Check sheet for the modelled part. Datum: model origin and axes. Units: mm. Face numbers are marked on the shaded views. A direction names the side the tool comes from. Round coordinates to 2 decimals unless told otherwise and drop trailing zeros. Loops run counter-clockwise (first coordinate to the right, second up) from the corner with the lowest first, then second, coordinate; pieces in that order, holes last. Notation, with made-up numbers: M 32.25,-32 L 59.25,-32 A6 ccw 59.25,-28 Z; hole C -22,-33.75 d10. An arc over 180 degrees is marked long. Write item = value, one per line. Start each with the question number.
(1) Go/stop test with flat-tipped pins: P1, Ø3, axis at y = 5, z = 1, coming from the -X side; P2, Ø3, axis at x = -18, z = 1, coming from the +Y side; P3, Ø2, axis at x = -126, z = 2.5, coming from the -Y side. Record where each tip stops, or that it passes through.
(2) Scan lines: L1, parallel to Y at x = -99.5, z = 12; L2, parallel to Z at x = -132, y = 28; L3, parallel to Y at x = -140, z = 0.9. Record each from-to range of solid material in increasing order. Write a range as from..to.
(3) Set-up check for the marked faces 1 and 2: record each of +Z, -Z, +X, -X, +Y, -Y from which the full face is reachable in a straight line by a thin tool's end or side.
(4) Mould release check, pull along X, two halves, no side actions. Record for the marked faces 3 and 4: pulls with the +X half, pulls with the -X half, needs draft (parallel to the pull), parting line crosses it, or undercut.
(5) Cross-section at A-A on x = -72.5. Record the boundary of the cut face in (y, z), plus the area to 3 significant figures.
(6) Cross-section at B-B on x = -127. Record the boundary of the cut face in (y, z).
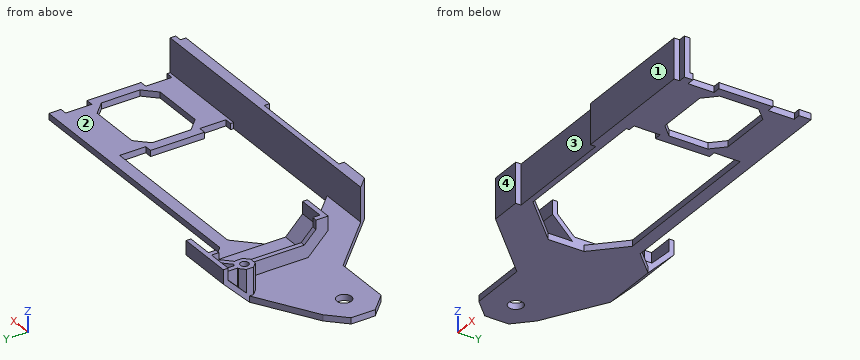
from build123d import *

# Parameters (mm, degrees)
SKETCH4_R            = 3
MAIN_WALL_DEPTH      = 2.5
BASE_DEPTH           = 14
BOSS_EXTRUDE8_DEPTH  = 2
BOSS_EXTRUDE9_DEPTH  = 11
BOSS_EXTRUDE15_DEPTH = 12.5
BOSS_EXTRUDE13_REACH = 169.888
SKETCH19_R           = 1.7
CUT_EXTRUDE1_DEPTH   = 7


with BuildPart() as part:
    # Sketch4 → Main Wall (new body)
    with BuildSketch(Plane.XY):
        Polygon((-97, 59.3), (-113.5, 59.3), (-120.5, 59.3), (-144.970562748, 45), (-152, 37.970562748), (-152, 28.029437252), (-144.970562748, 21), (-135.029437252, 21), (-121, 21), (-95.5, -4.5), (-82.786796564, -4.5), (-82.786796564, -2.25), (-35.786796564, -2.25), (-35.786796564, -4.5), (17, -4.5), (17, -2.25), (20, -2.25), (20, 1.25), (17, 1.25), (17, 12), (20, 12), (20, 34.25), (17, 34.25), (17, 45), (20, 45), (20, 50), (-87.7, 50), align=None)
        with Locations((-140, 33)):
            Circle(SKETCH4_R, mode=Mode.SUBTRACT)
        Polygon((-20, 0), (-20, 1.25), (-17, 1.25), (-17, 12), (-20, 12), (-20, 34.25), (-17, 34.25), (-17, 45), (-85, 45), (-97, 33), (-97, 18.213203436), (-78.786796564, 0), align=None, mode=Mode.SUBTRACT)
        Polygon((11, 36), (-11, 36), (-16, 31), (-16, 15), (-11, 10), (11, 10), (16, 15), (16, 31), align=None, mode=Mode.SUBTRACT)
    extrude(amount=MAIN_WALL_DEPTH)

    # Sketch5 → Base (add)
    with BuildSketch(Plane.XY.offset(2.5)):
        Polygon((20, 0), (20, -2.25), (17, -2.25), (17, -4.5), (-35.786796564, -4.5), (-35.786796564, -2.25), (-82.786796564, -2.25), (-82.786796564, -4.5), (-95.5, -4.5), (-100, 0), align=None)
    extrude(amount=BASE_DEPTH)

    # Sketch15 → Boss-Extrude8 (add)
    with BuildSketch(Plane(origin=(-108, 0, 0), x_dir=(0, 0, -1), z_dir=(1, 0, 0))):
        Polygon((0, 30.701010127), (0, 59.298989873), (-10.701010127, 70), (-16.5, 70), (-16.5, 68), (-16.5, 65), (-12.772077939, 65), (-8, 60.227922061), (-8, 29.772077939), (-12.772077939, 25), (-16.5, 25), (-16.5, 20), (-10.701010127, 20), align=None)
    extrude(amount=-BOSS_EXTRUDE8_DEPTH)

    # Sketch16 → Boss-Extrude9 (add)
    with BuildSketch(Plane(origin=(-108, 0, 0), x_dir=(0, 0, -1), z_dir=(1, 0, 0))):
        Polygon((-16.5, 68), (-11.529437252, 68), (-4.5, 60.970562748), (-4.5, 29.029437252), (-11.529437252, 22), (-16.5, 22), (-16.5, 20), (-10.701010127, 20), (0, 30.701010127), (0, 59.298989873), (-10.701010127, 70), (-16.5, 70), align=None)
    extrude(amount=BOSS_EXTRUDE9_DEPTH)

    # Sketch17 → Boss-Extrude15 (add)
    with BuildSketch(Plane(origin=(-108, 0, 0), x_dir=(0, 0, -1), z_dir=(1, 0, 0))):
        Polygon((0, 59.298989873), (-10.701010127, 70), (-16.5, 70), (-16.5, 68), (-11.529437252, 68), (-2.5, 58.970562748), (-2.5, 50), (0, 50), align=None)
    extrude(amount=-BOSS_EXTRUDE15_DEPTH)

    # Sketch18 → Boss-Extrude13 (add, up to next)
    with BuildSketch(Plane.XY.offset(13.5), mode=Mode.PRIVATE) as boss_extrude13_sk1:
        Polygon((-115.550252532, 62.5), (-116, 62.5), (-116, 69.5), (-118, 69.5), (-118, 62.5), (-118.449747468, 62.5), (-120.5, 60.449747468), (-120.5, 57.550252532), (-118.449747468, 55.5), (-115.550252532, 55.5), (-113.5, 57.550252532), (-113.5, 60.449747468), (-113.818019485, 60.767766953), (-108.161165235, 66.424621202), (-109.575378798, 67.838834765), (-115.232233047, 62.181980515), align=None)
    boss_extrude13_tool1 = extrude(boss_extrude13_sk1.sketch, amount=-BOSS_EXTRUDE13_REACH, mode=Mode.PRIVATE) - part.part
    add(boss_extrude13_tool1.solids().sort_by_distance((-115.797998, 61.590243, 13.5))[0])

    # Sketch19 → Cut-Extrude1 (cut)
    with BuildSketch(Plane.XY.offset(13.5)):
        with Locations((-117, 59)):
            Circle(SKETCH19_R)
    extrude(amount=-CUT_EXTRUDE1_DEPTH, mode=Mode.SUBTRACT)


solid = part.part
Result:
q1.P1 = -106.5
q1.P2 = 50
q1.P3 = 21
q2.L1 = -0.5..0, 20..22, 68..70
q2.L2 = 0..2.5
q2.L3 = 21..30, 36..47.9
q3.face_1 = +Z, -Z, +X, -X, -Y
q3.face_2 = +Z, +X, +Y
q4.face_3 = undercut
q4.face_4 = needs draft
q5.outline = M -2.25,0 L 0,0 L 0,16.5 L -2.25,16.5 Z; M 45,0 L 50,0 L 50,2.5 L 45,2.5 Z
q5.area = 49.6 mm^2
q6.outline = M 21,0 L 55.5,0 L 55.5,2.5 L 21,2.5 Z
